Source: CAD feature listing. Evaluate the final solid. Frame: model axes, mm. Coordinates: 2 decimals unless noted, no trailing zeros. Write each loop counter-clockwise with the first axis right and the second up, starting at its lowest first coordinate (ties: lowest second). Pieces come first, ordered by that corner, then holes. Notation, with made-up numbers: M -40,56 L -11,56 A20 ccw -11,73 Z; hole C 18.5,-33 d3. An arc over 180 degrees is marked long. One line per item, written item: value. Start each with the question number.
Item 1: Cut plane C-C, the plane x = 125. Output: boundary loops of the cut face in (y, z).
Item 2: Cut plane B-B, the plane y = 3.4. Output: boundary loops of the cut face in (x, z), then the cut area to 3 significant figures.
Item 3: Pin query (flat end, axial travel): P1, Ø1.5, axis at x = -17, y = 3.5, coming from the +Z side; P2, Ø12, axis at x = -62.5, z = -108.25, coming from the +Y side; P3, Ø1, axis at x = 48.5, y = 2, coming from the +Z side. Return the tip coordinate at first contact, or that it passes through.
Item 4: Ray query, L1, parallel to Z at x = -62.5, y = 4.8; L2, parallel to Z at x = 125, y = 3.4; L3, parallel to Z at x = -128.5, y = 0.7. Return the intervals inside material, ascending. Write a range as from..to.
Item 5: Cut plane A-A, the plane z = 0. Output: boundary loops of the cut face in (x, y), then the cut area to 3 significant figures.
Item 6: Cut plane D-D, the plane x = -62.5. Output: boundary loops of the cut face in (y, z), then the cut area to 3 significant figures.
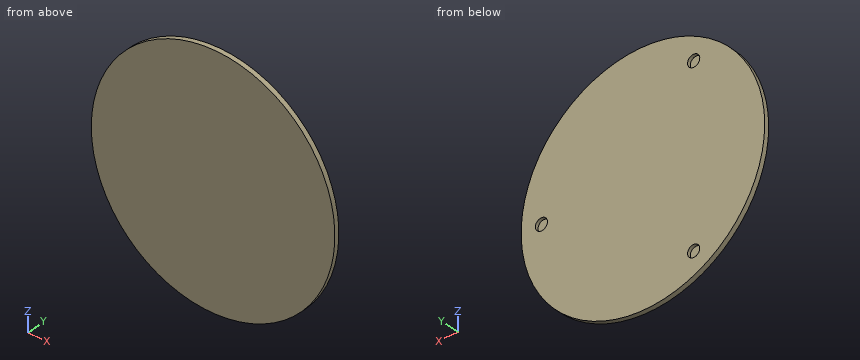
Autodesk Inventor part; units mm, degrees
ref_plane "YZ Plane" through (0, 0, 0) normal (1, 0, 0) x (0, 1, 0)
ref_plane "XZ Plane" through (0, 0, 0) normal (0, 1, 0) x (-1, 0, 0)
ref_plane "XY Plane" through (0, 0, 0) normal (0, 0, 1) x (1, 0, 0)
sketch "Sketch6" plane through (0, 0, 0) normal (0, 1, 0) x (-1, 0, 0)
  circle A0 centre (0, 0) radius 150
  dimension "d17" = 300
extrude "Extrusion3" add sketch "Sketch6" along normal blind 6
sketch "Sketch7" plane through (0, 6, 0) normal (0, 1, 0) x (1, 0, 0)
  circle A0 centre (0, 0) radius 125
  line L0 (125, 0) -> (-62.5, 108.2532) construction
  line L1 (-62.5, 108.2532) -> (-62.5, -108.2532) construction
  line L2 (-62.5, -108.2532) -> (125, 0) construction
  line L3 (0, 0) -> (125, 0) construction
  line L4 (-62.5, -108.2532) -> (0, 0) construction
  line L5 (0, 0) -> (-62.5, 108.2532) construction
  dimension "d20" = 250
hole "Hole2" at (125, 6, 0) direction (0, -1, 0) diameter 15 depth 4
hole "Hole3" at (-62.5, 6, 108.2532) direction (0, -1, 0) diameter 15 depth 4
hole "Hole4" at (-62.5, 6, -108.2532) direction (0, -1, 0) diameter 15 depth 4
properties part number "Fußßß"
From the geometry:
1. outline: M 0,-82.92 L 6,-82.92 L 6,-7.5 L 2,-7.5 L 2,7.5 L 6,7.5 L 6,82.92 L 0,82.92 Z
2. outline: C 0,0 d300; hole C -62.5,-108.25 d15; hole C -62.5,108.25 d15; hole C 125,0 d15
2. area: 70,200 mm²
3. P1: stops at z = 149.12
3. P2: stops at y = 2
3. P3: stops at z = 142.11
4. L1: z = -136.36..-115.75, -100.75..100.75, 115.75..136.36
4. L2: z = -82.92..-7.5, 7.5..82.92
4. L3: z = -77.38..77.38
5. outline: M -150,0 L 150,0 L 150,6 L 132.5,6 L 132.5,2 L 117.5,2 L 117.5,6 L -150,6 Z
5. area: 1,740 mm²
6. outline: M 0,-136.36 L 6,-136.36 L 6,-115.75 L 2,-115.75 L 2,-100.75 L 6,-100.75 L 6,100.75 L 2,100.75 L 2,115.75 L 6,115.75 L 6,136.36 L 0,136.36 Z
6. area: 1,520 mm²
